from build123d import *

# Parameters (mm, degrees)
F0_W     = 11.648168
F0_H     = 22.549662
F0_R     = 1.2065
F2_DEPTH = 6.35
F3_D     = 3.175
F5_D     = 3.175


with BuildPart() as f2:
    # F0 (on Top) → F2 (new body)
    with BuildSketch(Plane.XY):
        Rectangle(F0_W, F0_H)
        with Locations((0, -6.35)):
            Circle(F0_R, mode=Mode.SUBTRACT)
        with Locations((0, 6.35)):
            Circle(F0_R, mode=Mode.SUBTRACT)
    extrude(amount=F2_DEPTH)

    # F3 (through all)
    with Locations(Plane(origin=(0, 0, 0), x_dir=(0, 1, 0), z_dir=(-1, 0, 0))):
        with Locations((0, 0)):
            Hole(F3_D / 2)

    # F5 (through all)
    with Locations(Plane.YZ):
        with Locations((0, 0)):
            Hole(F5_D / 2)


solid = f2.part
Read the model definition and answer for the solid it produces. Units are mm, in the model's axes. Coordinates: 2 decimals unless noted, no trailing zeros. Write each loop counter-clockwise with the first axis right and the second up, starting at its lowest first coordinate (ties: lowest second). Pieces come first, ordered by that corner, then holes. Notation, with made-up numbers: (-37, 53) - (18, 53) arc R25 cw to (18, 92) - close; hole circle Ø5 at (-27.5, 53.25). An arc over 180 degrees is marked (long way). One line per question, with ' | ' between items.
Q1. Consider L1, parallel to Y at x = 0, z = 2.5; L2, parallel to Y at x = 0.25, z = 4.25; L3, parallel to X at y = 6.5, z = 3. Determine where each line is inside the solid, lowest interval first. Write a range as [from, to].
Result set:
L1: [-11.27, -7.56], [-5.14, 5.14], [7.56, 11.27] | L2: [-11.27, -7.53], [-5.17, 5.17], [7.53, 11.27] | L3: [-5.82, -1.2], [1.2, 5.82]
Q2. Determine the mould class of faces 1 (the cylindrical face through (-0.26, 5.17, 3.13)), 2 (the flat face through (-5.824, 0, 3)), 3 (the flat face through (0, -11.275, 3)) for opening direction Y: +Y half, -Y half, draft (parallel to the pull), parting line (faces both ways), or undercut.
Result set:
face 1: undercut | face 2: draft | face 3: -Y half
Q3. Find section C-C, the plane z = 2. Write down the section's boundary in (x, y).
Result set:
outline: (-5.82, -11.27) - (5.82, -11.27) - (5.82, 11.27) - (-5.82, 11.27) - close; hole circle Ø2.41 at (0, -6.35); hole circle Ø2.41 at (0, 6.35)
Q4. Find section A-A, the plane y = 6.35. Write down the section's boundary in (x, z), plus the area to 3 significant figures.
Result set:
outline: (-5.82, 0) - (-1.21, 0) - (-1.21, 6.35) - (-5.82, 6.35) - close; (1.21, 0) - (5.82, 0) - (5.82, 6.35) - (1.21, 6.35) - close | area: 58.6 mm^2
Q5. Find section B-B, the plane x = 0. State how many separate pieces and enclosed holes the cut face has, plus the area to 3 significant figures.
Result set:
separate pieces: 3 | enclosed holes: 0 | area: 109 mm^2
